Source: CAD feature listing. Evaluate the final solid. Frame: model axes, mm. A direction names the side the tool comes from. Give positions to 0.01 mm unless a question says otherwise; leave off trailing zeros. Order: outer loops, then holes, each group sorted by start corner. A loop starts at its lowest first (then second) coordinate and runs counter-clockwise, first axis right, second up.
1) Section D-D, the plane x = 0.5. Return loops of the section in (y, z).
2) Material intervals for line 1 (Y direction, x = 5, z = 0); line 2 (Y direction, x = 2.75, z = 0.7); line 3 (X direction, y = 6.75, z = -1.05), sorted ascending.
3) First-contact query: P1, Ø1, axis at y = 6.5, z = 0, coming from the +X side; P2, Ø0.6, axis at y = 6.5, z = 1, coming from the -X side. Flat tips, straight axial feed; report the tip coordinate or a pass-through.
4) Access query for faces 4 (the face through (0, 0, 0)), 5 (the face through (1, 7, 0)). Directions: +Z, -Z, +X, -X, +Y, -Y. A direction counts if a zero-diameter tool reaches every point of the face in a straight line with its end or side. Return the directions, or none.
5) Section B-B, the plane y = 6.75. Return loops of the section in (x, z).
6) Section C-C, the plane x = 4.5. Return loops of the section in (y, z), plus the area to 3 significant figures.
7) Section A-A, the plane z = 0. Return loops of the section in (x, y).
8) Draft query along Z for faces 1 (the face through (-1, 7, 0)), 2 (the face through (0, 13.5, 0)), 3 (the face through (5.56, 7.74, 0.13)). Return one class per face: released by +Z, released by -Z, zero draft, split by the parting line, or undercut.
```python
from build123d import *

# Parameters (mm, degrees)
SKETCH_1_R           = 1
EXTRUDE_1_DEPTH      = 13.5
SKETCH_4_R           = 1.5
EXTRUDE_3_DEPTH      = 10
SKETCH_7_R           = 1
CUT_EXTRUDE_15_DEPTH = 9


with BuildPart() as part:
    # Sketch 1 → Extrude 1 (new body)
    with BuildSketch(Plane(origin=(0, 0, 0), x_dir=(1, 0, 0), z_dir=(0, 1, 0))):
        with Locations(Location((0, 0, 0), (0, 0, 270))):
            Circle(SKETCH_1_R)
    extrude(amount=EXTRUDE_1_DEPTH)

    # Sketch 4 → Extrude 3 (add)
    with BuildSketch(Plane(origin=(0, 0, 0), x_dir=(0, 0, -1), z_dir=(1, 0, 0))):
        with Locations(Location((0, 6.75, 0), (0, 0, 228.189685104))):
            Circle(SKETCH_4_R)
    extrude(amount=EXTRUDE_3_DEPTH)

    # Sketch 7 → Cut-Extrude 15 (cut)
    with BuildSketch(Plane(origin=(10, 0, 0), x_dir=(0, 0, -1), z_dir=(1, 0, 0))):
        with Locations((0, 6.75)):
            Circle(SKETCH_7_R)
    extrude(amount=-CUT_EXTRUDE_15_DEPTH, mode=Mode.SUBTRACT)


solid = part.part
```
From the geometry:
1. outline: (0, -0.87) - (5.53, -0.87) arc R1.5 ccw to (7.97, -0.87) - (13.5, -0.87) - (13.5, 0.87) - (7.97, 0.87) arc R1.5 ccw to (5.53, 0.87) - (0, 0.87) - close
2. line 1: y = 5.25 to 5.75, 7.75 to 8.25
2. line 2: y = 5.42 to 6.04, 7.46 to 8.08
2. line 3: x = 0 to 10
3. P1: stops at x = 1
3. P2: stops at x = -0.71
4. face 4: +Z, -Z, +X, -X, -Y
4. face 5: +X
5. outline: (0, -1.5) - (10, -1.5) - (10, -1) - (1, -1) - (1, 1) - (10, 1) - (10, 1.5) - (0, 1.5) - (0, 1) arc R1 ccw to (0, -1) - close
6. outline: circle Ø3 at (6.75, 0); hole circle Ø2 at (6.75, 0)
6. area: 3.93 mm2
7. outline: (-1, 0) - (1, 0) - (1, 5.25) - (10, 5.25) - (10, 5.75) - (1, 5.75) - (1, 7.75) - (10, 7.75) - (10, 8.25) - (1, 8.25) - (1, 13.5) - (-1, 13.5) - close
8. face 1: split by the parting line
8. face 2: zero draft
8. face 3: undercut
